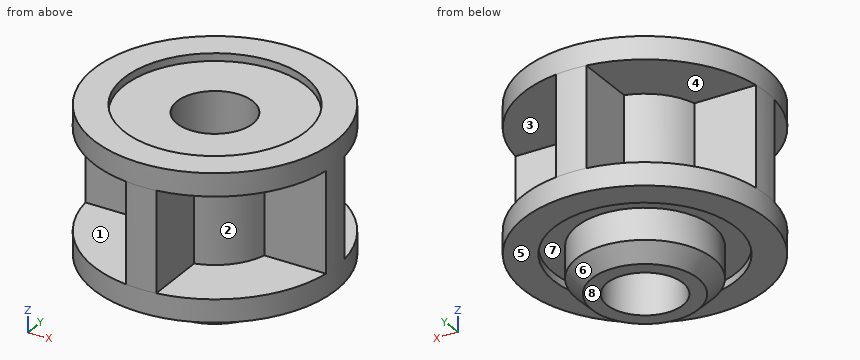
```python
from build123d import *

# Parameters (mm, degrees)
F0_R             = 12.7
F0_R_2           = 3.96875
F1_DEPTH         = 1.5875
F2_R             = 12.7
F2_R_2           = 9.525
F3_DEPTH         = 0.79375
F4_R             = 6.35
F4_R_2           = 3.96875
F5_DEPTH         = 10.4694736
F6_R             = 12.7
F6_R_2           = 3.96875
F7_DEPTH         = 1.5875
F8_R             = 12.7
F8_R_2           = 9.525
F9_DEPTH         = 0.79375
F11_DEPTH        = 10.4694736
F11_COPIES_COUNT = 4
F12_R            = 7.14375
F12_R_2          = 3.96875
F13_DEPTH        = 4.85775
F14_SIZE         = 1.5875


# Not quite as in the source:
# - a length typed as a fraction of an inch, garbled in the dataset ("3 / 203.2 mm" for 3/8 in), is restored
# - a pattern or mirror of a feature is missing from the dataset's text; its kind, count and spacing are read off the source's solid


with BuildPart() as f1:
    # F0 (on Top) → F1 (new body)
    with BuildSketch(Plane.XY):
        Circle(F0_R)
        Circle(F0_R_2, mode=Mode.SUBTRACT)
    extrude(amount=F1_DEPTH)

    # F2 (on face) → F3 (join)
    with BuildSketch(Plane(origin=(0, 0, 0), x_dir=(1, 0, 0), z_dir=(0, 0, -1))):
        Circle(F2_R)
        Circle(F2_R_2, mode=Mode.SUBTRACT)
    extrude(amount=F3_DEPTH)

    # F4 (on face) → F5 (join)
    with BuildSketch(Plane.XY.offset(1.5875)):
        Circle(F4_R)
        Circle(F4_R_2, mode=Mode.SUBTRACT)
    extrude(amount=F5_DEPTH)

    # F6 (on face) → F7 (join)
    with BuildSketch(Plane.XY.offset(12.0569736)):
        Circle(F6_R)
        Circle(F6_R_2, mode=Mode.SUBTRACT)
    extrude(amount=F7_DEPTH)

    # F8 (on face) → F9 (join)
    with BuildSketch(Plane.XY.offset(13.6444736)):
        Circle(F8_R)
        Circle(F8_R_2, mode=Mode.SUBTRACT)
    extrude(amount=F9_DEPTH)

    # F10 (on face) → F11 (join, through all)
    with BuildSketch(Plane.XY.offset(1.5875)):
        with BuildLine():
            Line((1.5875, -12.6003906189), (1.5875, -6.1483610621))
            ThreePointArc((1.5875, -6.1483610621), (0, -6.35), (-1.5875, -6.1483610621))
            Line((-1.5875, -6.1483610621), (-1.5875, -12.6003906189))
            ThreePointArc((-1.5875, -12.6003906189), (0, -12.7), (1.5875, -12.6003906189))
        make_face()
    f11 = extrude(amount=F11_DEPTH)

    # F11_copies: F11 ×4 about axis
    f11_copies_axis = Axis((0, 0, 0), (0, 0, 1))
    for i in range(1, F11_COPIES_COUNT):
        add(f11.rotate(f11_copies_axis, i * 360 / F11_COPIES_COUNT))

    # F12 (on face) → F13 (join)
    with BuildSketch(Plane(origin=(0, 0, 0), x_dir=(1, 0, 0), z_dir=(0, 0, -1))):
        Circle(F12_R)
        Circle(F12_R_2, mode=Mode.SUBTRACT)
    extrude(amount=F13_DEPTH)

    # F14
    f14_edges = [f1.edges().sort_by_distance(p)[0] for p in [
        (-7.14375, 0, -4.85775),
    ]]
    chamfer(f14_edges, length=F14_SIZE)


solid = f1.part
```
Design review of the part built by this model. Coordinates are the model's own, in mm. Face numbers are marked on the shaded views. A direction names the side the tool comes from. Coordinates: 2 decimals unless noted, no trailing zeros. Write each loop counter-clockwise with the first axis right and the second up, starting at its lowest first coordinate (ties: lowest second). Pieces come first, ordered by that corner, then holes.
1) Add section A-A (x = 0). Write out the cut boundary in (y, z) (1 decimal), plus the area to 3 significant figures.
2) Machinability: for the marked faces 1, 2, 3, 4 and 5, which of the approach directions +Z, -Z, +X, -X, +Y, -Y give a long, thin tool a straight path to every point of the face, cutting with its end or side? Answer none if there is none.
3) To check wall thickness, follow L1, parallel to X at y = 0, z = -0.15 (3 decimals); L2, parallel to Z at x = 3, y = 11.5; L3, parallel to X at y = 0, z = 7. State the ranges of each line that lie inside material, in increasing order.
4) Add section D-D (y = 8.5). Write out the cut boundary in (x, z).
5) Mouldability with a two-part tool opening along X and no side actions: class the marked faces 6, 7 and 8 as +X half, -X half, draft (parallel to the pull), parting line (faces both ways), or undercut.
6) Add section C-C (z = 11.25). Write out the cut boundary in (x, y).
7) Insertion check: pin 1 (5.5 mm diameter, centred on x = -2.5, y = -3, fed in from +Z); pin 2 (1.5 mm diameter, centred on x = -4.5, z = 2.5, fed in from -Y); pin 3 (5.5 mm diameter, centred on x = 6.5, y = -9, fed in from -Z). Each pin has a flat end and moves straight along its axis. Give the tip position at first contact, or say it passes through.
Check result:
1. outline: (-12.7, -0.8) - (-9.5, -0.8) - (-9.5, 0) - (-7.1, 0) - (-7.1, -3.3) - (-5.6, -4.9) - (-4, -4.9) - (-4, 13.6) - (-9.5, 13.6) - (-9.5, 14.4) - (-12.7, 14.4) - close; (4, -4.9) - (5.6, -4.9) - (7.1, -3.3) - (7.1, 0) - (9.5, 0) - (9.5, -0.8) - (12.7, -0.8) - (12.7, 14.4) - (9.5, 14.4) - (9.5, 13.6) - (4, 13.6) - close
1. area: 277 mm2
2. face 1: -X, -Y
2. face 2: +X, -Y
2. face 3: +X, +Y
2. face 4: -X, +Y
2. face 5: -Z
3. L1: x = -12.7 to -9.525, -7.144 to -3.969, 3.969 to 7.144, 9.525 to 12.7
3. L2: z = -0.79 to 1.59, 12.06 to 14.44
3. L3: x = -12.7 to -3.97, 3.97 to 12.7
4. outline: (-9.44, -0.79) - (-4.3, -0.79) - (-4.3, 0) - (4.3, 0) - (4.3, -0.79) - (9.44, -0.79) - (9.44, 1.59) - (1.59, 1.59) - (1.59, 12.06) - (9.44, 12.06) - (9.44, 14.44) - (4.3, 14.44) - (4.3, 13.64) - (-4.3, 13.64) - (-4.3, 14.44) - (-9.44, 14.44) - (-9.44, 12.06) - (-1.59, 12.06) - (-1.59, 1.59) - (-9.44, 1.59) - close
5. face 6: parting line
5. face 7: undercut
5. face 8: draft
6. outline: (-12.6, -1.59) - (-6.15, -1.59) arc R6.35 ccw to (-1.59, -6.15) - (-1.59, -12.6) arc R12.7 ccw to (1.59, -12.6) - (1.59, -6.15) arc R6.35 ccw to (6.15, -1.59) - (12.6, -1.59) arc R12.7 ccw to (12.6, 1.59) - (6.15, 1.59) arc R6.35 ccw to (1.59, 6.15) - (1.59, 12.6) arc R12.7 ccw to (-1.59, 12.6) - (-1.59, 6.15) arc R6.35 ccw to (-6.15, 1.59) - (-12.6, 1.59) arc R12.7 ccw to start; hole circle Ø7.94 at (0, 0)
7. pin 1: stops at z = 13.64
7. pin 2: stops at y = -5.12
7. pin 3: stops at z = -0.79
